Build history of the part. All positions in model axes, mm. A direction names the side the tool comes from. Give positions to 0.01 mm unless a question says otherwise; leave off trailing zeros. Loops run counter-clockwise (first coordinate to the right, second up) from the corner with the lowest first, then second, coordinate; pieces in that order, holes last. Notation, with made-up numbers: (-3.75, 75) - (19.25, 75) arc R21 cw to (19.25, 85) - close; hole circle Ø11 at (86.25, 1). An arc over 180 degrees is marked (long way). Return JSON: item names as keys, results as strings. Group by question number.
1) 3-axis set-ups, long thin cutter, end or side, ignore diameter. For faces 1 (the face through (15.5, 77, 2)), 2 (the face through (-8, 33, 5)), 3 (the face through (76, 12.4, 3)): which of +Z, -Z, +X, -X, +Y, -Y reach the whole face in a straight line?
2) Slice it at B-B (x = -5). List the corners of the cut face in (y, z).
3) Mould opens along Y. For faces 4 (the face through (74.16, 34.09, 2.54)), 5 (the face through (-5, 12.4, 2)), 6 (the face through (81, 32, 3)) say: released by +Y, released by -Y, zero draft, split by the parting line, or undercut.
4) Drop flat-ended pins along their axis: pin 1 (4 mm diameter, centred on x = 76.5, z = 2.5, fed in from +Y); pin 2 (1.5 mm diameter, centred on x = 63, z = 6, fed in from +Y); pin 3 (5.5 mm diameter, centred on x = -3.5, z = 3, fed in from -Y). Give the stop position or say it passes through.
5) Drill centre lines: probe 1 along Y at (x, z) = (35.5, 8.4); probe 2 along Y at (x, z) = (35.5, 2.05); probe 3 along X at (y, z) = (31, 6.75). Where is each one in solid material? Low to high. Write a range as from..to.
6) Slice it at A-A (y = 77.4). List the corners of the cut face in (x, z).
7) Slice it at C-C (z = 2.5). List the corners of the cut face in (x, y), and give its area (3 significant figures).
8) Slice it at D-D (x = 35.5). List the corners of the cut face in (y, z).
Autodesk Inventor part; units mm, degrees
ref_plane "YZ Plane" through (0, 0, 0) normal (1, 0, 0) x (0, 1, 0)
ref_plane "XZ Plane" through (0, 0, 0) normal (0, 1, 0) x (-1, 0, 0)
ref_plane "XY Plane" through (0, 0, 0) normal (0, 0, 1) x (1, 0, 0)
sketch "Sketch1" plane through (0, 0, 0) normal (0, 0, 1) x (1, 0, 0)
  line L0 (0, 0) -> (71, 0)
  line L1 (71, 0) -> (71, 72.4)
  line L2 (71, 72.4) -> (0, 72.4)
  line L3 (0, 72.4) -> (0, 0)
  dimension "d0" = 71
  dimension "d1" = 72.4
extrude "Extrusion1" add sketch "Sketch1" along normal blind 10
sketch "Sketch2" plane through (0, 0, 10) normal (0, 0, 1) x (1, 0, 0)
  line L0 (71, 0) -> (71, 72.4)
  line L1 (71, 12.4) -> (81, 12.4)
  line L2 (81, 12.4) -> (81, 52.4)
  line L3 (81, 52.4) -> (71, 52.4)
  line L4 (71, 52.4) -> (71, 12.4)
  line L5 (71, 72.4) -> (0, 72.4)
  circle A0 centre (76, 32.4) radius 2.5
  line L6 (0, 0) -> (71, 0)
  point P0 (81, 32.4)
  point P1 (76, 52.4)
  dimension "d4" = 10
  dimension "d5" = 40
  dimension "d7" = 5
  dimension "d53" = 20
extrude "Extrusion2" add sketch "Sketch2" against normal blind 10
sketch "Sketch3" plane through (0, 0, 10) normal (0, 0, 1) x (1, 0, 0)
  line L0 (71, 52.4) -> (81, 52.4)
  line L1 (71, 12.4) -> (81, 12.4)
  line L2 (81, 52.4) -> (71, 52.4)
  line L3 (71, 52.4) -> (71, 12.4)
  line L4 (71, 12.4) -> (81, 12.4)
  line L5 (81, 12.4) -> (81, 52.4)
  point P0 (0, 0)
extrude "Extrusion3" cut sketch "Sketch3" against normal blind 5
sketch "Sketch8" plane through (0, 0, 0) normal (0, 0, -1) x (-1, 0, 0)
  line L0 (-15.5, 10) -> (-55.5, 10)
  line L1 (-55.5, 10) -> (-55.5, 0)
  line L2 (-55.5, 0) -> (-15.5, 0)
  line L3 (-15.5, 0) -> (-15.5, 10)
  line L4 (0, 0) -> (-71, 0)
  line L5 (-71, 0) -> (-71, 12.4)
  line L6 (-71, 72.4) -> (0, 72.4)
  point P0 (-35.5, 0)
  point P1 (-35.5, 0)
  point P2 (-35.5, 10)
  point P3 (-35.5, 72.4)
  dimension "d32" = 40
  dimension "d33" = 10
extrude "Extrusion8" cut sketch "Sketch8" against normal blind 5
sketch "Sketch9" plane through (0, 0, 5) normal (0, 0, -1) x (-1, 0, 0)
  line L0 (-55.5, 0) -> (-55.5, 10) construction
  line L1 (-15.5, 10) -> (-15.5, 0) construction
  circle A0 centre (-35.5, 5) radius 2.5
  line L2 (-55.5, 10) -> (-15.5, 10)
  line L3 (-15.5, 0) -> (-55.5, 0)
  point P0 (0, 0)
  point P1 (-35.5, 0)
  point P2 (-15.5, 5)
  dimension "d37" = 5
extrude "Extrusion9" cut sketch "Sketch9" against normal through all
sketch "Sketch10" plane through (0, 0, 0) normal (0, 0, -1) x (-1, 0, 0)
  line L0 (0, 72.4) -> (0, 0)
  line L1 (0, 12.4) -> (10, 12.4)
  line L2 (10, 12.4) -> (10, 52.4)
  line L3 (10, 52.4) -> (0, 52.4)
  line L4 (0, 52.4) -> (0, 12.4)
  circle A0 centre (5, 32.4) radius 2.5
  point P0 (-81, 12.4)
  point P1 (10, 32.4)
  point P2 (5, 12.4)
  dimension "d40" = 10
  dimension "d41" = 40
  dimension "d42" = 5
extrude "Extrusion10" add sketch "Sketch10" against normal blind 5
sketch "Sketch11" plane through (0, 0, 0) normal (0, 0, -1) x (-1, 0, 0)
  line L0 (-71, 72.4) -> (0, 72.4)
  line L1 (-15.5, 72.4) -> (-55.5, 72.4)
  line L2 (-55.5, 72.4) -> (-55.5, 82.4)
  line L3 (-55.5, 82.4) -> (-15.5, 82.4)
  line L4 (-15.5, 82.4) -> (-15.5, 72.4)
  circle A0 centre (-35.5, 77.4) radius 2.5
  point P0 (0, 0)
  point P1 (-35.5, 82.4)
  point P2 (-35.5, 72.4)
  point P3 (-15.5, 77.4)
  dimension "d46" = 40
  dimension "d47" = 10
  dimension "d48" = 5
extrude "Extrusion11" add sketch "Sketch11" against normal blind 5
properties part number "SP002" material "ABS Plastic"
Results:
{
 "1": {"face 1": "+Z, -Z, -X, +Y", "face 2": "+Z, -X, +Y, -Y", "face 3": "+Z, -Z, +X, -Y"},
 "2": {"outline": "(12.4, 0) - (29.9, 0) - (29.9, 5) - (12.4, 5) - close; (34.9, 0) - (52.4, 0) - (52.4, 5) - (34.9, 5) - close"},
 "3": {"face 4": "undercut", "face 5": "released by -Y", "face 6": "zero draft"},
 "4": {"pin 1": "y = 52.4", "pin 2": "y = 72.4", "pin 3": "y = 12.4"},
 "5": {"probe 1": "0..2.5, 7.5..72.4", "probe 2": "10..74.9, 79.9..82.4", "probe 3": "0..71"},
 "6": {"outline": "(15.5, 0) - (33, 0) - (33, 5) - (15.5, 5) - close; (38, 0) - (55.5, 0) - (55.5, 5) - (38, 5) - close"},
 "7": {"outline": "(-10, 12.4) - (0, 12.4) - (0, 0) - (15.5, 0) - (15.5, 10) - (55.5, 10) - (55.5, 0) - (71, 0) - (71, 12.4) - (81, 12.4) - (81, 52.4) - (71, 52.4) - (71, 72.4) - (55.5, 72.4) - (55.5, 82.4) - (15.5, 82.4) - (15.5, 72.4) - (0, 72.4) - (0, 52.4) - (-10, 52.4) - close; hole circle Ø5 at (-5, 32.4); hole circle Ø5 at (35.5, 77.4); hole circle Ø5 at (76, 32.4)", "area": "5,880 mm2"},
 "8": {"outline": "(0, 5) - (2.5, 5) - (2.5, 10) - (0, 10) - close; (7.5, 5) - (10, 5) - (10, 0) - (74.9, 0) - (74.9, 5) - (72.4, 5) - (72.4, 10) - (7.5, 10) - close; (79.9, 0) - (82.4, 0) - (82.4, 5) - (79.9, 5) - close"}
}
